Can you work these out from the drawing? Everything is in mm from the part's minimum corner. Round coordinates to 2 decimals unless told otherwise and drop trailing zeros. Write each loop counter-clockwise with the first axis right and the second up, starting at its lowest first coordinate (ties: lowest second). Pieces come first, ordered by that corner, then holes. Notation, with made-up numbers: M 58,73 L 105,73 A32 ccw 105,100 Z; hole C -11.75,-11.75 d1. An arc over 180 degrees is marked long. Use a Markdown table: item, result. Add a question column.
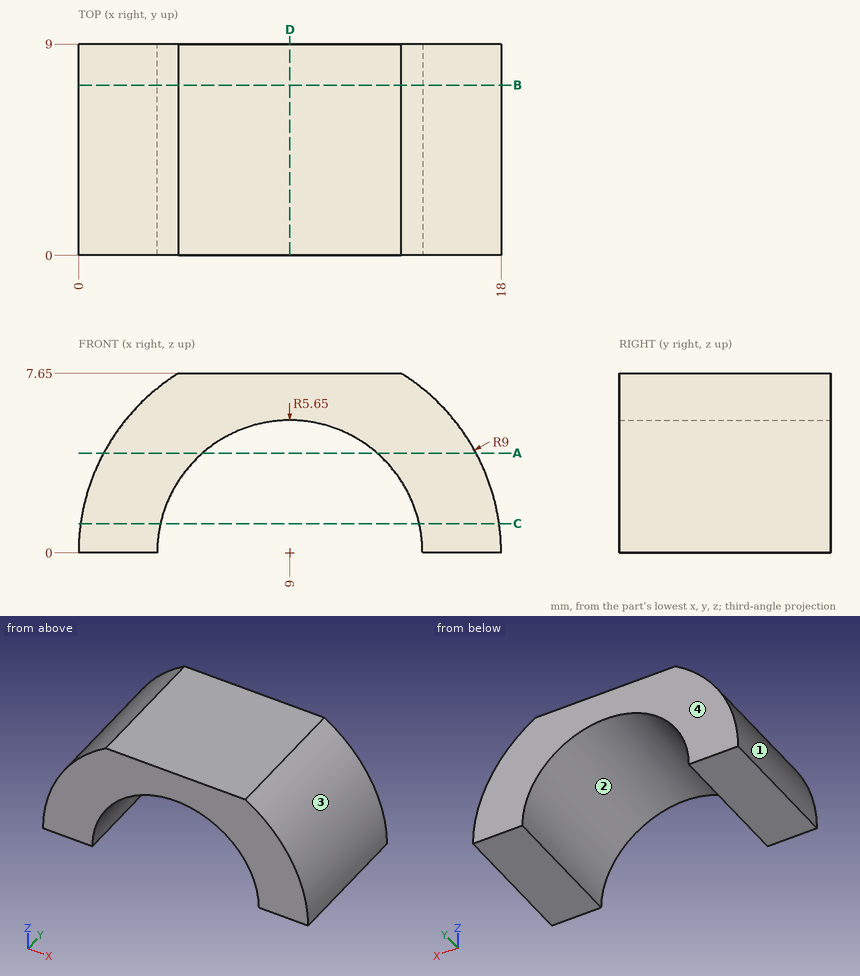
Item 1: For pin 1 Ø2 at (y, z) = (2.5, 4) entering from +X; pin 2 Ø1 at (y, z) = (7, 1.5) entering from +X; pin 3 Ø3 at (y, z) = (6, 5.5) entering from -X, each with a flat end and sliding along its axis, tell me the tip position at first contact or that it passes through.
Item 2: Imagine slicing it at B-B on y = 7.25. List the corners of the cut face in (x, z) for me, plus the area to 3 significant figures.
Item 3: I need wall thicknesses on probe 1 along X at (y, z) = (8.5, 5); probe 2 along X at (y, z) = (3, 2); probe 3 along Z at (x, y) = (6.5, 0.5). Which ranges of each line are inside material? Lowest first, please. Write a range as from..to.
Item 4: Imagine slicing it at A-A on z = 4.25. List the corners of the cut face in (x, y) for me.
Item 5: If we mould it in two halves opening along X, with no side actions, what happens to the marked faces 1, 2, 3 and 4? For each: +X half, -X half, draft (parallel to the pull), parting line (faces both ways), or undercut.
Item 6: Imagine slicing it at D-D on x = 9. List the corners of the cut face in (y, z) for me, plus the area to 3 significant figures.
Item 7: Imagine slicing it at C-C on z = 1.25. List the corners of the cut face in (x, y) for me, plus the area to 4 significant figures.
The answers:
| question | item | result |
|---|---|---|
| 1 | pin 1 | x = 17.49 |
| 1 | pin 2 | x = 17.94 |
| 1 | pin 3 | x = 0.94 |
| 2 | outline | M 0,0 L 3.35,0 A5.65 cw 14.65,0 L 18,0 A9 ccw 13.74,7.65 L 4.26,7.65 A9 ccw Z |
| 2 | area | 68.4 mm² |
| 3 | probe 1 | 1.52..6.37, 11.63..16.48 |
| 3 | probe 2 | 0.23..3.72, 14.28..17.77 |
| 3 | probe 3 | 5.07..7.65 |
| 4 | outline | M 1.07,0 L 5.28,0 L 5.28,9 L 1.07,9 Z; M 12.72,0 L 16.93,0 L 16.93,9 L 12.72,9 Z |
| 5 | face 1 | -X half |
| 5 | face 2 | undercut |
| 5 | face 3 | +X half |
| 5 | face 4 | draft |
| 6 | outline | M 0,5.65 L 9,5.65 L 9,7.65 L 0,7.65 Z |
| 6 | area | 18.0 mm² |
| 7 | outline | M 0.09,0 L 3.49,0 L 3.49,9 L 0.09,9 Z; M 14.51,0 L 17.91,0 L 17.91,9 L 14.51,9 Z |
| 7 | area | 61.25 mm² |
